from build123d import *

# Parameters (mm, degrees)
SKETCH1_R             = 33.655
BOSS_EXTRUDE1_DEPTH   = 4.7625
SKETCH2_W             = 50.3
SKETCH2_H             = 41.3
BOSS_EXTRUDE2_DEPTH   = 31.7
F_6_CLEARANCE_HOLE1_D = 3.7973
SKETCH6_W             = 44.3
SKETCH6_H             = 35.3
CUT_EXTRUDE1_DEPTH    = 28.7
SKETCH7_W             = 32
SKETCH7_H             = 14
CUT_EXTRUDE2_DEPTH    = 3
FILLET1_R             = 1.5
CUT_EXTRUDE3_DEPTH    = 70.334846623
MIRROR2_COPY_1_DEPTH  = 70.334846623


with BuildPart() as part:
    # Sketch1 → Boss-Extrude1 (new body)
    with BuildSketch(Plane(origin=(0, 0, 0), x_dir=(1, 0, 0), z_dir=(0, 1, 0))):
        with Locations(Location((0, 0, 0), (0, 0, 90))):
            Circle(SKETCH1_R)
    extrude(amount=BOSS_EXTRUDE1_DEPTH)

    # Sketch2 → Boss-Extrude2 (add)
    with BuildSketch(Plane(origin=(0, 4.7625, 0), x_dir=(1, 0, 0), z_dir=(0, 1, 0))):
        Rectangle(SKETCH2_W, SKETCH2_H)
    extrude(amount=-BOSS_EXTRUDE2_DEPTH)

    # #6 Clearance Hole1 (through all)
    with Locations(Plane(origin=(0, 4.7625, 0), x_dir=(1, 0, 0), z_dir=(0, 1, 0))):
        with Locations((0, 29.5275), (29.5275, 0), (0, -29.5275), (-29.5275, 0)):
            Hole(F_6_CLEARANCE_HOLE1_D / 2)

    # Sketch6 → Cut-Extrude1 (cut)
    with BuildSketch(Plane(origin=(0, 4.7625, 0), x_dir=(1, 0, 0), z_dir=(0, 1, 0))):
        Rectangle(SKETCH6_W, SKETCH6_H)
    cut_extrude1 = extrude(amount=-CUT_EXTRUDE1_DEPTH, mode=Mode.SUBTRACT)

    # Sketch7 → Cut-Extrude2 (cut)
    with BuildSketch(Plane(origin=(25.15, 0, 0), x_dir=(0, 0, -1), z_dir=(1, 0, 0))):
        with Locations((0, -15.9375)):
            Rectangle(SKETCH7_W, SKETCH7_H)
    extrude(amount=-CUT_EXTRUDE2_DEPTH, mode=Mode.SUBTRACT)

    # Fillet1
    fillet1_edges = [part.edges().sort_by_distance(p)[0] for p in [
        (25.15, -13.46875, 20.65),
        (-25.15, -26.9375, 0),
        (-25.15, -13.46875, 20.65),
        (0, -26.9375, -20.65),
        (-25.15, -13.46875, -20.65),
        (0, 0, -20.65),
        (-25.15, 0, 0),
        (0, 0, 20.65),
        (25.15, 0, 0),
        (25.15, -26.9375, 0),
        (25.15, -13.46875, -20.65),
        (0, -26.9375, 20.65),
    ]]
    fillet(fillet1_edges, radius=FILLET1_R)

    # Sketch14 → Cut-Extrude3 (cut, through all)
    with BuildSketch(Plane.XY.offset(-20.65)):
        with BuildLine():
            Line((13.3, -8.4375), (13.3, -4.4375))
            ThreePointArc((13.3, -4.4375), (15, -2.7375), (16.7, -4.4375))
            Line((16.7, -4.4375), (16.7, -8.4375))
            ThreePointArc((16.7, -8.4375), (15, -10.1375), (13.3, -8.4375))
        make_face()
    cut_extrude3 = extrude(amount=CUT_EXTRUDE3_DEPTH, mode=Mode.SUBTRACT)

    # Mirror1: Cut-Extrude3 across plane
    add(cut_extrude3.mirror(Plane(origin=(0, 0, 0), x_dir=(0, 0, 1), z_dir=(1, 0, 0))), mode=Mode.SUBTRACT)

    # Mirror2: Cut-Extrude1, Cut-Extrude3 across plane
    add(cut_extrude1.mirror(Plane.ZX.offset(-13.4375)), mode=Mode.SUBTRACT)
    add(cut_extrude3.mirror(Plane.ZX.offset(-13.4375)), mode=Mode.SUBTRACT)

    # Mirror2 copy 1 sketch → Mirror2 copy 1 (cut, through all)
    with BuildSketch(Plane(origin=(0, -26.875, -20.65), x_dir=(-1, 0, 0), z_dir=(0, 0, 1))):
        with BuildLine():
            Line((13.3, -8.4375), (13.3, -4.4375))
            ThreePointArc((13.3, -4.4375), (15, -2.7375), (16.7, -4.4375))
            Line((16.7, -4.4375), (16.7, -8.4375))
            ThreePointArc((16.7, -8.4375), (15, -10.1375), (13.3, -8.4375))
        make_face()
    extrude(amount=MIRROR2_COPY_1_DEPTH, mode=Mode.SUBTRACT)


solid = part.part
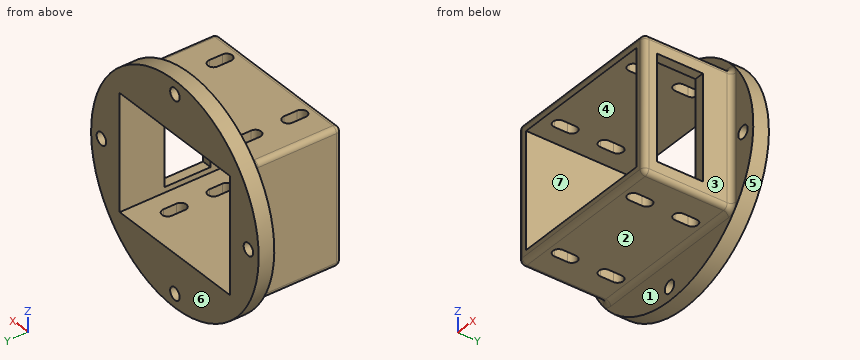
Build history of the part. All positions in model axes, mm. Face numbers are marked on the shaded views. A direction names the side the tool comes from. Round coordinates to 2 decimals unless told otherwise and drop trailing zeros. Loops run counter-clockwise (first coordinate to the right, second up) from the corner with the lowest first, then second, coordinate; pieces in that order, holes last. Notation, with made-up numbers: (73, 49) -> (120, 49) arc R11 ccw to (120, 59) -> close; hole circle Ø11 at (15.25, -21.5). An arc over 180 degrees is marked (long way). Answer in a Markdown table with one row per item.
Item 1: Saw through at C-C (y = -12.5). Write the cut outline in (x, z), and give its area (3 significant figures).
Answers below:
| item | result |
|---|---|
| outline | (-25.15, -19.15) arc R1.5 ccw to (-23.65, -20.65) -> (23.65, -20.65) arc R1.5 ccw to (25.15, -19.15) -> (25.15, -16) -> (22.15, -16) -> (22.15, -17.65) -> (-22.15, -17.65) -> (-22.15, 17.65) -> (22.15, 17.65) -> (22.15, 16) -> (25.15, 16) -> (25.15, 19.15) arc R1.5 ccw to (23.65, 20.65) -> (-23.65, 20.65) arc R1.5 ccw to (-25.15, 19.15) -> close |
| area | 416 mm² |
Item 2: Drill centre lines: L1, parallel to Z at x = -21, y = -8; L2, parallel to X at y = -8, z = 10; L3, parallel to Y at x = 23.5, z = -2. Where is each one in solid material? Low to high. Write a range as [from, to].
Answers below:
| item | result |
|---|---|
| L1 | z = [-20.65, -17.65], [17.65, 20.65] |
| L2 | x = [-25.15, -22.15], [22.15, 25.15] |
| L3 | y = [-26.94, -22.94], [-8.94, 4.76] |
Item 3: Mould opens along Z. For the marked faces 4, 5, 6 and 7 say: +Z half, -Z half, draft (parallel to the pull), parting line (faces both ways), or undercut.
Answers below:
| item | result |
|---|---|
| face 4 | undercut |
| face 5 | parting line |
| face 6 | draft |
| face 7 | undercut |
Item 4: Saw through at A-A (z = 0). State how many separate pieces and enclosed holes the cut face has, and give its area (3 significant figures).
Answers below:
| item | result |
|---|---|
| separate pieces | 5 |
| enclosed holes | 0 |
| area | 193 mm² |
Item 5: Which spindle directions (+Z, -Z, +X, -X, +Y, -Y) get a long thin tool onto all of the face, cutting with end or side? Do the marked faces 1, 2 and 3. Say none if no direction does.
Answers below:
| item | result |
|---|---|
| face 1 | -Y |
| face 2 | -Z, +X, -X, -Y |
| face 3 | +Z, -Z, +X, -Y |
Item 6: Saw through at D-D (z = 9.5). Write the cut outline in (x, y), and give its area (3 significant figures).
Answers below:
| item | result |
|---|---|
| outline | (-32.29, 0) -> (-26.65, 0) arc R1.5 cw to (-25.15, -1.5) -> (-25.15, -25.44) arc R1.5 ccw to (-23.65, -26.94) -> (-22.15, -26.94) -> (-22.15, 4.76) -> (-32.29, 4.76) -> close; (22.15, -26.94) -> (23.65, -26.94) arc R1.5 ccw to (25.15, -25.44) -> (25.15, -22.94) -> (22.15, -22.94) -> close; (22.15, -8.94) -> (25.15, -8.94) -> (25.15, -1.5) arc R1.5 cw to (26.65, 0) -> (32.29, 0) -> (32.29, 4.76) -> (22.15, 4.76) -> close |
| area | 216 mm² |
Item 7: Pin check, flat tips, straight feed: pin 1 (3.5 mm diameter, centred on y = -5.5, z = 18.5, fed in from +X); pin 2 (4 mm diameter, centred on x = 16.5, y = -22.5, fed in from +Z); pin 3 (12 mm diameter, centred on y = -14.5, z = 19, fed in from -X). Stop position of each tip, or through.
Answers below:
| item | result |
|---|---|
| pin 1 | stops at x = 25.15 |
| pin 2 | stops at z = 20.65 |
| pin 3 | stops at x = -25.15 |
